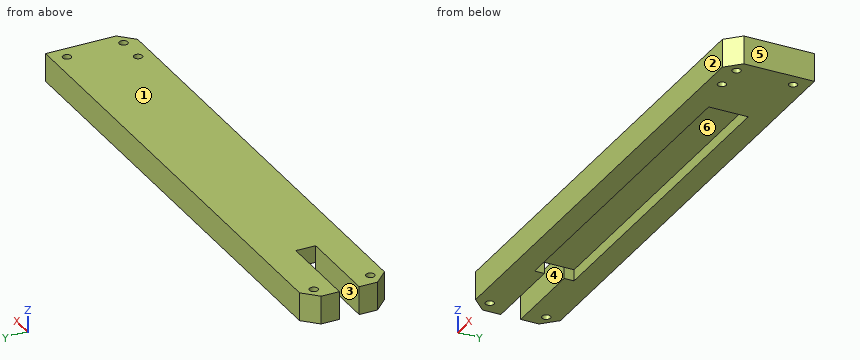
Autodesk Inventor part; units mm, degrees
ref_plane "YZ Plane" through (0, 0, 0) normal (1, 0, 0) x (0, 1, 0)
ref_plane "XZ Plane" through (0, 0, 0) normal (0, 1, 0) x (-1, 0, 0)
ref_plane "XY Plane" through (0, 0, 0) normal (0, 0, 1) x (1, 0, 0)
sketch "Sketch1" plane through (0, 0, 0) normal (0, 0, 1) x (1, 0, 0)
  line L0 (-109.7802, 23.5714) -> (70.2198, 23.5714)
  line L1 (70.2198, 23.5714) -> (70.2198, -6.4286)
  line L2 (70.2198, -6.4286) -> (-109.7802, -6.4286)
  line L3 (-109.7802, -6.4286) -> (-109.7802, 23.5714)
  point P0 (0, 0)
  dimension "d0" = 180
  dimension "d1" = 30
extrude "Extrusion1" add sketch "Sketch1" along normal blind 10
sketch "Sketch2" plane through (0, 0, 10) normal (0, 0, 1) x (1, 0, 0)
  line L0 (-109.7802, 23.5714) -> (-109.7802, -6.4286)
  line L1 (-109.7802, -6.4286) -> (70.2198, -6.4286)
  line L2 (70.2198, 23.5714) -> (-109.7802, 23.5714)
  point P0 (0, 0)
  point P1 (-104.7802, 18.5714)
  point P2 (-104.7802, -1.4286)
  dimension "d4" = 5
  dimension "d5" = 5
  dimension "d6" = 5
  dimension "d7" = 5
hole "Hole1" at (-104.7802, 18.5714, 10) at (-104.7802, -1.4286, 10) direction (0, 0, -1) diameter 3 depth 10 tip angle 118
chamfer "Chamfer1" distance 5 angle 45 2 edges at (-109.7802, 23.5714, 5) (-109.7802, -6.4286, 5)
sketch "Sketch3" plane through (0, 0, 0) normal (0, 0, -1) x (-1, 0, 0)
  line L0 (109.7802, 18.5714) -> (109.7802, -1.4286)
  line L1 (109.7802, 12.0714) -> (79.7802, 12.0714)
  line L2 (79.7802, 12.0714) -> (79.7802, 5.0714)
  line L3 (79.7802, 5.0714) -> (109.7802, 5.0714)
  line L4 (109.7802, 5.0714) -> (109.7802, 12.0714)
  circle A0 centre (104.7802, 18.5714) radius 1.5
  circle A1 centre (104.7802, -1.4286) radius 1.5
  point P0 (0, 0)
  dimension "d18" = 5
  dimension "d19" = 5
  dimension "d20" = 30
extrude "Extrusion2" cut sketch "Sketch3" against normal blind 10 contours L0 L3 L2 L1
sketch "Sketch4" plane through (0, 0, 0) normal (0, 0, -1) x (-1, 0, 0)
  line L0 (-40.2198, 15.5714) -> (79.7802, 15.5714)
  line L1 (79.7802, 15.5714) -> (79.7802, 1.5714)
  line L2 (79.7802, 1.5714) -> (-40.2198, 1.5714)
  line L3 (-40.2198, 1.5714) -> (-40.2198, 15.5714)
  line L4 (-70.2198, 23.5714) -> (104.7802, 23.5714)
  line L5 (-70.2198, -6.4286) -> (104.7802, -6.4286)
  line L6 (79.7802, 5.0714) -> (79.7802, 12.0714)
  line L7 (-70.2198, 23.5714) -> (-70.2198, -6.4286)
  point P0 (0, 0)
  dimension "d23" = 8
  dimension "d24" = 8
  dimension "d25" = 30
extrude "Extrusion3" cut sketch "Sketch4" against normal blind 4
sketch "Sketch5" plane through (0, 0, 0) normal (0, 0, -1) x (-1, 0, 0)
  line L0 (104.7802, 23.5714) -> (-70.2198, 23.5714)
  line L1 (-70.2198, -6.4286) -> (104.7802, -6.4286)
  line L2 (-70.2198, 23.5714) -> (-70.2198, -6.4286)
  point P0 (0, 0)
  point P1 (-65.2198, 18.5714)
  point P2 (-65.2198, -1.4286)
  point P3 (-55.2198, -1.4286)
  dimension "d28" = 5
  dimension "d29" = 5
  dimension "d30" = 5
  dimension "d31" = 5
  dimension "d32" = 5
  dimension "d33" = 10
hole "Hole2" at (65.2198, 18.5714, 0) at (65.2198, -1.4286, 0) at (55.2198, -1.4286, 0) direction (0, 0, 1) diameter 3 depth 10 tip angle 118
chamfer "Chamfer2" distance 5 angle 45 1 edges at (70.2198, -6.4286, 5)
properties part number "Connection Bar"
For this review, take the finished solid that the model builds, in its own axes (mm). Face numbers are marked on the shaded views. A direction names the side the tool comes from. Round coordinates to 2 decimals unless told otherwise and drop trailing zeros. Write each loop counter-clockwise with the first axis right and the second up, starting at its lowest first coordinate (ties: lowest second). Pieces come first, ordered by that corner, then holes. Notation, with made-up numbers: (7.25, 83.25) -> (22.25, 83.25) arc R35 ccw to (22.25, 122.25) -> close; hole circle Ø11 at (4, 8.5). An arc over 180 degrees is marked (long way). One line per question, with ' | ' between items. Start each with the question number.
(1) For line 1 along Y through (x, z) = (-96, 5.25); line 2 along Y through (x, z) = (-22.5, 3.75); line 3 along X through (y, z) = (-1, 6.25), list the stretches that pass through material, from the lowest coordinate up. Write a range as from..to.
(2) Insertion check: P1, Ø4, axis at x = 3.5, y = 9, coming from the -Z side; P2, Ø3, axis at y = 7, z = 8.5, coming from the -X side. Each pin has a flat end and moves straight along its axis. Give the tip position at first contact, or say it passes through.
(3) Add section A-A, the plane z = 1.75. Write out the cut boundary in (x, y), plus the area to 3 significant figures.
(4) Tool access review of the marked faces 4, 5 and 6: name each direction out of +Z, -Z, +X, -X, +Y, -Y from which nothing blocks a thin tool from reaching the whole face with its end or side.
(5) Add section D-D, the plane z = 8.25. Write out the cut boundary in (x, y), plus the area to 3 significant figures.
(6) Add section C-C, the plane y = 14. Write out the cut boundary in (x, z), plus the area to 3 significant figures.
(7) Add section B-B, the plane x = -48. Write out the cut boundary in (y, z), plus the area to 3 significant figures.
(8) Mouldability with a two-part tool opening along Y and no side actions: class the marked faces 1, 2 and 3 as released by +Y, released by -Y, zero draft, split by the parting line, or undercut.
Answer list:
1) line 1: -6.43..5.07, 12.07..23.57 | line 2: -6.43..1.57, 15.57..23.57 | line 3: -109.78..-106.22, -103.34..53.78, 56.66..63.78, 66.66..70.22
2) P1: z = 4 | P2: x = -79.78
3) outline: (-109.78, -1.43) -> (-104.78, -6.43) -> (65.22, -6.43) -> (70.22, -1.43) -> (70.22, 23.57) -> (-104.78, 23.57) -> (-109.78, 18.57) -> (-109.78, 12.07) -> (-79.78, 12.07) -> (-79.78, 15.57) -> (40.22, 15.57) -> (40.22, 1.57) -> (-79.78, 1.57) -> (-79.78, 5.07) -> (-109.78, 5.07) -> close; hole circle Ø3 at (-104.78, -1.43); hole circle Ø3 at (-104.78, 18.57); hole circle Ø3 at (55.22, -1.43); hole circle Ø3 at (65.22, -1.43); hole circle Ø3 at (65.22, 18.57) | area: 3,440 mm²
4) face 4: +Z, -Z, -X | face 5: +Z, -Z, +X, +Y, -Y | face 6: -Z
5) outline: (-109.78, -1.43) -> (-104.78, -6.43) -> (65.22, -6.43) -> (70.22, -1.43) -> (70.22, 23.57) -> (-104.78, 23.57) -> (-109.78, 18.57) -> (-109.78, 12.07) -> (-79.78, 12.07) -> (-79.78, 5.07) -> (-109.78, 5.07) -> close; hole circle Ø3 at (-104.78, -1.43); hole circle Ø3 at (-104.78, 18.57); hole circle Ø3 at (55.22, -1.43); hole circle Ø3 at (65.22, -1.43); hole circle Ø3 at (65.22, 18.57) | area: 5,120 mm²
6) outline: (-109.78, 0) -> (-79.78, 0) -> (-79.78, 4) -> (40.22, 4) -> (40.22, 0) -> (70.22, 0) -> (70.22, 10) -> (-109.78, 10) -> close | area: 1,320 mm²
7) outline: (-6.43, 0) -> (1.57, 0) -> (1.57, 4) -> (15.57, 4) -> (15.57, 0) -> (23.57, 0) -> (23.57, 10) -> (-6.43, 10) -> close | area: 244 mm²
8) face 1: zero draft | face 2: released by -Y | face 3: undercut
